Design review of the part built by this model. Coordinates are the model's own, in mm. A direction names the side the tool comes from. Coordinates: 2 decimals unless noted, no trailing zeros. Write each loop counter-clockwise with the first axis right and the second up, starting at its lowest first coordinate (ties: lowest second). Pieces come first, ordered by that corner, then holes.
Q1. Take a section at C-C, the plane z = 0.85. State how many separate pieces and enclosed holes the cut face has, plus the area to 3 significant figures.
Q2. Take a section at B-B, the plane y = 0.5. Write out the cut boundary in (x, z).
Q3. For faces 3 (the cylindrical face through (20.036, 95.052, 1.479)), 4 (the flat face through (39.659, -34, 1)), 5 (the cylindrical face through (49.773, -48.313, 1.479)), 6 (the cylindrical face through (18.6, 46.04, 1.48)), list the 3-axis set-ups (+Z, -Z, +X, -X, +Y, -Y) from which the entire face can be reached by the end or side of a thin tool; tool diameter is ignored.
Q4. Take a section at A-A, the plane y = -30.5. Write out the cut boundary in (x, z).
Q5. For L1, parallel to X at y = -5, z = 0.25; L2, parallel to X at y = 66, z = 0.6; L3, parallel to X at y = 20, z = 0.4, list the stretches that pass through material, from the lowest coordinate up.
Q6. For pin 1 Ø1.5 at (y, z) = (-34.5, 1.5) entering from +X; pin 2 Ø0.9 at (x, z) = (27.5, 2) entering from +Y; pin 3 Ø0.9 at (y, z) = (-34.5, 1.5) entering from +X; pin 4 Ø2 at (x, y) = (52.5, 46.5) entering from -Z, all flat-tipped, find the tip position at first contact; note any pin that passes through.
Q7. The part is to be moulded in two halves that separate along Y. For faces 1 (the flat face through (20.659, -34, 1)), 2 (the cylindrical face through (48.852, 94.935, 1.479)), say which applies: released by +Y, released by -Y, zero draft, split by the parting line, or undercut.
from build123d import *

# Parameters (mm, degrees)
MODEL_R                 = 8
MODEL_W                 = 8.2
MODEL_H                 = 3
SALIENTE_EXTRUIR1_DEPTH = 3


with BuildPart() as part:
    # Model → Saliente-Extruir1 (new body)
    with BuildSketch(Plane.XY):
        with BuildLine():
            Line((53.481445034, 31.38247243), (46.779993349, 33.353487631))
            ThreePointArc((46.779993349, 33.353487631), (45.927013388, 33.861110925), (45.423137443, 34.716309882))
            Line((45.423137443, 34.716309882), (43.357228049, 40.767605918))
            ThreePointArc((43.357228049, 40.767605918), (49.8242529, 45.957956881), (55.030233707, 52.412406306))
            ThreePointArc((55.030233707, 52.412406306), (61.093598066, 69.288732485), (58.730938319, 87.064913502))
            ThreePointArc((58.730938319, 87.064913502), (57.207808393, 89.703172008), (54.961022773, 91.760424326))
            ThreePointArc((54.961022773, 91.760424326), (48.760554591, 94.970135555), (41.983416035, 96.648958014))
            ThreePointArc((41.983416035, 96.648958014), (34.455707931, 97.499868783), (26.92255254, 96.698614587))
            ThreePointArc((26.92255254, 96.698614587), (19.94147438, 95.017139449), (13.543281779, 91.757393696))
            ThreePointArc((13.543281779, 91.757393696), (11.296797252, 89.699812596), (9.774053436, 87.061331216))
            ThreePointArc((9.774053436, 87.061331216), (7.413995161, 69.284804627), (13.479829214, 52.409365969))
            ThreePointArc((13.479829214, 52.409365969), (18.686734846, 45.955698119), (25.154492019, 40.766303923))
            Line((25.154492019, 40.766303923), (23.089449249, 34.714697754))
            ThreePointArc((23.089449249, 34.714697754), (22.585696773, 33.859426062), (21.732790104, 33.351679631))
            Line((21.732790104, 33.351679631), (15.03162304, 31.379696979))
            ThreePointArc((15.03162304, 31.379696979), (14.337279285, 31.302558661), (13.658765154, 31.468938177))
            ThreePointArc((13.658765154, 31.468938177), (6.813868189, 30.682998994), (4.157550352, 24.325775512))
            ThreePointArc((4.157550352, 24.325775512), (3.052384752, 15.584544005), (3.445376772, 6.78249444))
            ThreePointArc((3.445376772, 6.78249444), (2.079974129, -1.555345588), (3.171410736, -9.933451987))
            ThreePointArc((3.171410736, -9.933451987), (2.64421566, -13.051552622), (2.238579914, -16.187783777))
            ThreePointArc((2.238579914, -16.187783777), (2.76704769, -17.326785827), (3.90620228, -17.854924712))
            ThreePointArc((3.90620228, -17.854924712), (7.260899106, -18.072090773), (10.49984033, -17.171862116))
            ThreePointArc((10.49984033, -17.171862116), (10.811965124, -16.338126213), (10.499599615, -15.504480466))
            ThreePointArc((10.499599615, -15.504480466), (11.162118239, -14.900674558), (11.484662699, -14.0643268))
            ThreePointArc((11.484662699, -14.0643268), (10.631367301, -12.166232415), (9.28624721, -10.578300657))
            ThreePointArc((9.28624721, -10.578300657), (8.805524833, -9.975430237), (8.452370377, -9.289989739))
            ThreePointArc((8.452370377, -9.289989739), (9.932418252, -2.08907189), (9.895592327, 5.262281961))
            ThreePointArc((9.895592327, 5.262281961), (11.66577443, 9.648300332), (12.584225099, 14.288036336))
            ThreePointArc((12.584225099, 14.288036336), (13.262246612, 0.566960759), (16.497509918, -12.784469858))
            ThreePointArc((16.497509918, -12.784469858), (16.042177417, -24.524016518), (18.211841217, -36.070307803))
            ThreePointArc((18.211841217, -36.070307803), (18.02570309, -38.378850147), (18.612581504, -40.61929405))
            ThreePointArc((18.612581504, -40.61929405), (18.748290938, -48.20736643), (19.104485347, -55.78828887))
            ThreePointArc((19.104485347, -55.78828887), (15.202287094, -57.1012499), (11.634214393, -59.155483354))
            ThreePointArc((11.634214393, -59.155483354), (11.43855886, -59.470730285), (11.514005122, -59.834006456))
            ThreePointArc((11.514005122, -59.834006456), (12.025516155, -60.292514594), (12.695797103, -60.442836581))
            Line((12.695797103, -60.442836581), (22.259216422, -60.533409729))
            Line((22.259216422, -60.533409729), (22.259232154, -56.531748667))
            Line((22.259232154, -56.531748667), (25.259232154, -56.531748667))
            Line((25.259232154, -56.531748667), (25.259232342, -60.533048512))
            Line((25.259232342, -60.533048512), (29.098103748, -60.532494304))
            ThreePointArc((29.098103748, -60.532494304), (29.711184017, -60.322402882), (30.066706369, -59.780545262))
            ThreePointArc((30.066706369, -59.780545262), (31.946344773, -47.306061086), (31.46168815, -34.700074258))
            ThreePointArc((31.46168815, -34.700074258), (32.162582874, -23.89009615), (32.552547443, -13.064441077))
            ThreePointArc((32.552547443, -13.064441077), (34.246727454, -11.820907742), (35.966107002, -13.029359245))
            ThreePointArc((35.966107002, -13.029359245), (36.368868995, -23.871724918), (37.060905712, -34.699476107))
            ThreePointArc((37.060905712, -34.699476107), (36.577860738, -47.305611007), (38.45911007, -59.779939467))
            ThreePointArc((38.45911007, -59.779939467), (38.814710645, -60.321745755), (39.427821238, -60.531748667))
            Line((39.427821238, -60.531748667), (43.259232154, -60.531748667))
            Line((43.259232154, -60.531748667), (43.259232154, -56.531748667))
            Line((43.259232154, -56.531748667), (46.259232154, -56.531748667))
            Line((46.259232154, -56.531748667), (46.259232154, -60.531748667))
            Line((46.259232154, -60.531748667), (55.830114769, -60.439722986))
            ThreePointArc((55.830114769, -60.439722986), (56.500374008, -60.289304234), (57.011818842, -59.830722256))
            ThreePointArc((57.011818842, -59.830722256), (57.087212657, -59.467435196), (56.891511615, -59.152216515))
            ThreePointArc((56.891511615, -59.152216515), (53.335182459, -57.072918402), (49.420928579, -55.788560868))
            ThreePointArc((49.420928579, -55.788560868), (49.776142638, -48.206407611), (49.910836364, -40.617133427))
            ThreePointArc((49.910836364, -40.617133427), (50.497421978, -38.376559304), (50.310964473, -36.06799077))
            ThreePointArc((50.310964473, -36.06799077), (52.490190754, -24.554218645), (52.051420468, -12.844246127))
            ThreePointArc((52.051420468, -12.844246127), (54.289526358, 2.333645055), (55.635574328, 17.616499945))
            ThreePointArc((55.635574328, 17.616499945), (56.545662292, 11.300275423), (58.621246197, 5.265799159))
            ThreePointArc((58.621246197, 5.265799159), (58.585481568, -2.085559931), (60.066569006, -9.286264035))
            ThreePointArc((60.066569006, -9.286264035), (59.713513509, -9.97175551), (59.232878172, -10.574695324))
            ThreePointArc((59.232878172, -10.574695324), (57.88798734, -12.162821257), (57.034965974, -14.06103881))
            ThreePointArc((57.034965974, -14.06103881), (57.357631173, -14.897339994), (58.020236959, -15.50105025))
            ThreePointArc((58.020236959, -15.50105025), (57.707991805, -16.334741084), (58.020236959, -17.168431917))
            ThreePointArc((58.020236959, -17.168431917), (61.259308114, -18.068192968), (64.613973553, -17.850542599))
            ThreePointArc((64.613973553, -17.850542599), (65.753051885, -17.322239264), (66.28135522, -16.183160932))
            ThreePointArc((66.28135522, -16.183160932), (65.875266709, -13.04698837), (65.347621487, -9.928963878))
            ThreePointArc((65.347621487, -9.928963878), (66.437848557, -1.550699998), (65.071242216, 6.786942824))
            ThreePointArc((65.071242216, 6.786942824), (65.462963502, 15.589049032), (64.356535965, 24.330120898))
            ThreePointArc((64.356535965, 24.330120898), (61.699300379, 30.686960828), (54.854290022, 31.471911822))
            ThreePointArc((54.854290022, 31.471911822), (54.175799918, 31.305434353), (53.481445034, 31.38247243))
        make_face()
        with Locations((21.259232154, 70.846618638)):
            Circle(MODEL_R, mode=Mode.SUBTRACT)
        with Locations((47.259232154, 70.846618638)):
            Circle(MODEL_R, mode=Mode.SUBTRACT)
        Polygon((34.759232154, 26.002609393), (50.259232154, 26.002609393), (50.259232154, -5.997390607), (18.259232154, -5.997390607), (18.259232154, 26.002609393), (33.759232154, 26.002609393), align=None, mode=Mode.SUBTRACT)
        with Locations((24.759438839, -34.100057584)):
            Rectangle(MODEL_W, MODEL_H, mode=Mode.SUBTRACT)
        with Locations((43.759438839, -34.100057584)):
            Rectangle(MODEL_W, MODEL_H, mode=Mode.SUBTRACT)
    extrude(amount=SALIENTE_EXTRUIR1_DEPTH)


solid = part.part
Responses:
1. separate pieces: 1
1. enclosed holes: 5
1. area: 5,250 mm2
2. outline: (2.19, 0) - (10.09, 0) - (10.09, 3) - (2.19, 3) - close; (13.27, 0) - (18.26, 0) - (18.26, 3) - (13.27, 3) - close; (50.26, 0) - (54.07, 0) - (54.07, 3) - (50.26, 3) - close; (58.42, 0) - (66.33, 0) - (66.33, 3) - (58.42, 3) - close
3. face 3: +Z, -Z, -X, +Y
3. face 4: +Z, -Z
3. face 5: +Z, -Z, +X
3. face 6: +Z, -Z, -X
4. outline: (16.83, 0) - (31.77, 0) - (31.77, 3) - (16.83, 3) - close; (36.76, 0) - (51.7, 0) - (51.7, 3) - (36.76, 3) - close
5. L1: x = 2.23 to 9.52, 14.29 to 18.26, 50.26 to 53.32, 59 to 66.29
5. L2: x = 7.91 to 14.89, 27.62 to 40.89, 53.62 to 60.6
5. L3: x = 3.42 to 18.26, 50.26 to 65.09
6. pin 1: stops at x = 50.97
6. pin 2: stops at y = 96.91
6. pin 3: stops at x = 50.89
6. pin 4: passes through
7. face 1: undercut
7. face 2: released by +Y
